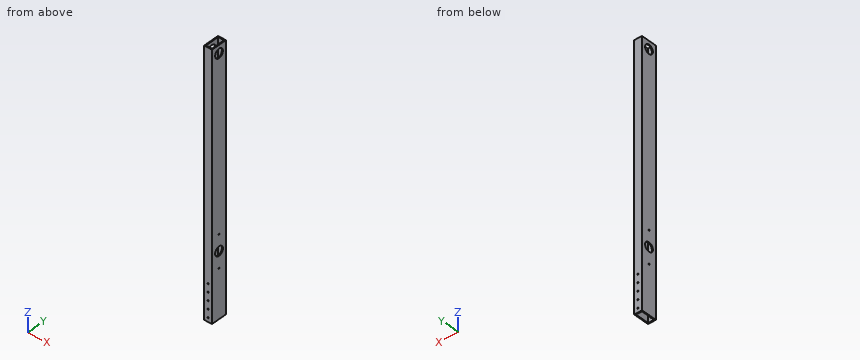
from build123d import *

# Parameters (mm, degrees)
SKETCH1_W           = 25.4
SKETCH1_H           = 50.8
SKETCH1_W_2         = 19.05
SKETCH1_H_2         = 44.45
BOSS_EXTRUDE1_DEPTH = 409.575
SKETCH7_R           = 1.905
CUT_EXTRUDE1_DEPTH  = 413.908719483
SKETCH8_R           = 1.905
SKETCH8_R_2         = 14.2875
CUT_EXTRUDE2_DEPTH  = 412.147176355


with BuildPart() as part:
    # Sketch1 → Boss-Extrude1 (new, symmetric)
    with BuildSketch(Plane.XY):
        Rectangle(SKETCH1_W, SKETCH1_H)
        Rectangle(SKETCH1_W_2, SKETCH1_H_2, mode=Mode.SUBTRACT)
    extrude(amount=BOSS_EXTRUDE1_DEPTH, both=True)

    # Sketch7 → Cut-Extrude1 (cut, through all)
    with BuildSketch(Plane(origin=(0, 25.4, 0), x_dir=(1, 0, 0), z_dir=(0, 1, 0))):
        with Locations(Location((0, 396.875, 0), (0, 0, 270))):
            Circle(SKETCH7_R)
        with Locations(Location((0, 371.475, 0), (0, 0, 270))):
            Circle(SKETCH7_R)
        with Locations(Location((0, 346.075, 0), (0, 0, 270))):
            Circle(SKETCH7_R)
        with Locations(Location((0, 320.675, 0), (0, 0, 270))):
            Circle(SKETCH7_R)
        with Locations(Location((0, 295.275, 0), (0, 0, 270))):
            Circle(SKETCH7_R)
    extrude(amount=-CUT_EXTRUDE1_DEPTH, mode=Mode.SUBTRACT)

    # Sketch8 → Cut-Extrude2 (cut, through all)
    with BuildSketch(Plane(origin=(12.7, 0, 0), x_dir=(0, 0, -1), z_dir=(1, 0, 0))):
        with Locations(Location((155.575, 0, 0), (0, 0, 90))):
            Circle(SKETCH8_R)
        with Locations(Location((257.175, 0, 0), (0, 0, 90))):
            Circle(SKETCH8_R)
        with Locations(Location((206.184267809, 0, 0), (0, 0, 90))):
            Circle(SKETCH8_R_2)
        with Locations(Location((-384.175, 0, 0), (0, 0, 90))):
            Circle(SKETCH8_R_2)
    extrude(amount=-CUT_EXTRUDE2_DEPTH, mode=Mode.SUBTRACT)


solid = part.part
Read the model definition and answer for the solid it produces. Units are mm, in the model's axes. Round coordinates to 2 decimals unless told otherwise and drop trailing zeros. Write each loop counter-clockwise with the first axis right and the second up, starting at its lowest first coordinate (ties: lowest second). Pieces come first, ordered by that corner, then holes.
1. The part is cut by section A-A, the plane z = -248.5. Determine the outline of the cut face in (x, y) (3 decimals).
2. Straight lines are drawn through the part: L1, parallel to Z at x = 11.9, y = 0 (1 decimal); L2, parallel to Y at x = 2.75, z = 307 (3 decimals); L3, parallel to X at y = 20.5, z = 157.5 (3 decimals). For each, find the intervals that lie inside material, in ascending order.
3. Given pin 1 Ø23 at (y, z) = (0, 384.175) entering from +X; pin 2 Ø5 at (x, z) = (0, -320.675) entering from +Y, each flat-ended and moving along its own axis, determine where each tip first touches the part or whether it passes through.
Values:
1. outline: (-12.7, -25.4) - (12.7, -25.4) - (12.7, 25.4) - (-12.7, 25.4) - close; hole (-9.525, -22.225) - (9.525, -22.225) - (9.525, 22.225) - (-9.525, 22.225) - close
2. L1: z = -409.6 to -259.1, -255.3 to -220.5, -191.9 to -157.5, -153.7 to 369.9, 398.5 to 409.6
2. L2: y = -25.4 to -22.225, 22.225 to 25.4
2. L3: x = -12.7 to -9.525, 9.525 to 12.7
3. pin 1: passes through
3. pin 2: stops at y = 25.4
